Verification items for this drawing (mm, ordinates from the low corner). Round coordinates to 2 decimals unless told otherwise and drop trailing zeros. Loops run counter-clockwise (first coordinate to the right, second up) from the corner with the lowest first, then second, coordinate; pieces in that order, holes last. Notation, with made-up numbers: (46.5, 66) -> (74.5, 66) arc R17 cw to (74.5, 93) -> close; hole circle Ø2 at (-20.5, -18.75). An arc over 180 degrees is marked (long way). Use a Markdown table: item, result. Add a question column.
Q1. Sectioned sample at B-B, the plane z = 27.5. Enter the section's corners in (x, y).
Q2. Release check for a two-part mould opening along X. For the marked faces 1 and 2 record: released by +X, released by -X, zero draft, split by the parting line, or undercut.
Q3. Sectioned sample at C-C, the plane y = 118. Enter the section's corners in (x, z).
Q4. Gauge pin test, flat ends, axial feed: P1, Ø2, axis at x = 7, z = 23.5, coming from the -Y side; P2, Ø1.5, axis at y = 126.5, z = 52.5, coming from the -X side; P3, Ø8, axis at x = 8.5, y = 47, coming from the +Z side; P4, Ø2.5, axis at x = 52.5, y = 125, coming from the +Z side. Record the tip position at first contact, or that the pin passes through.
Q5. Sectioned sample at A-A, the plane x = 27.5. Enter the section's corners in (y, z).
Q6. Material ranges on L1, parallel to X at y = 41.5, z = 27.5; L2, parallel to Z at x = 27, y = 59; L3, parallel to Z at x = 25, y = 42, recorded low to high.
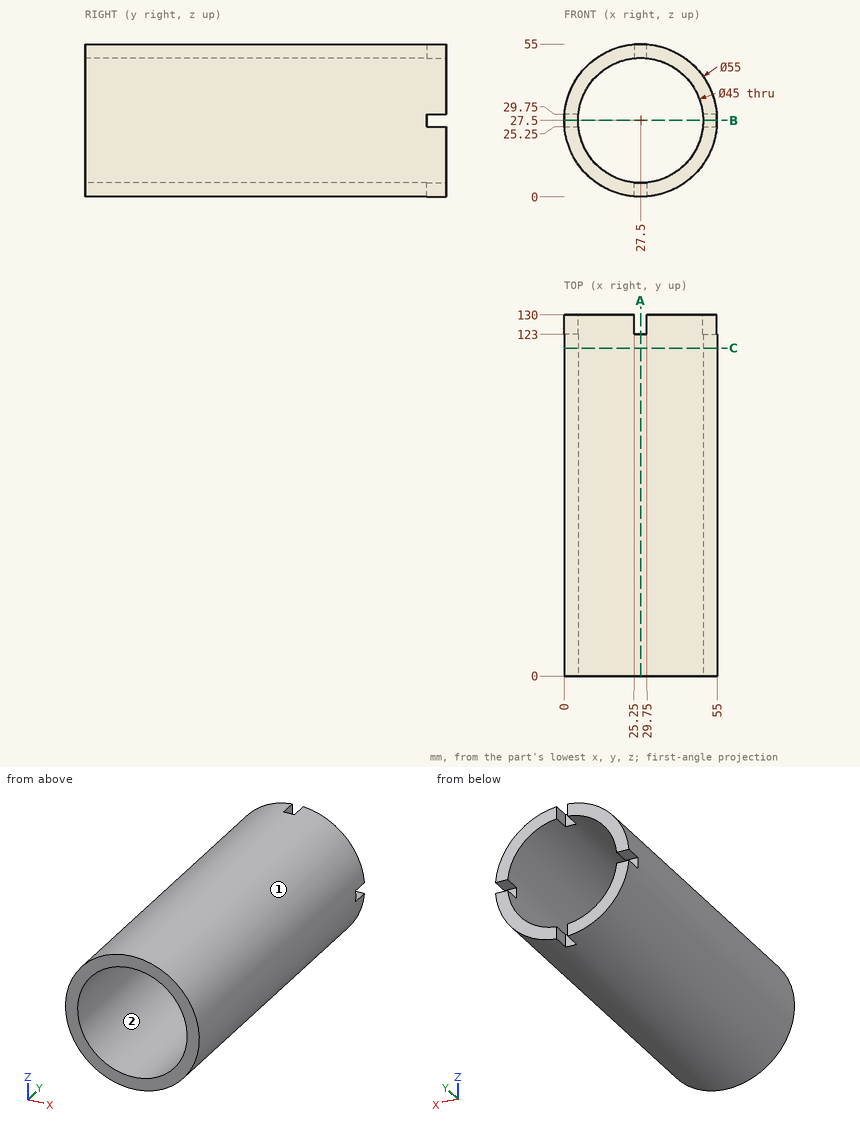
Values:
| question | item | result |
|---|---|---|
| 1 | outline | (0, 0) -> (5, 0) -> (5, 123) -> (0, 123) -> close; (50, 0) -> (55, 0) -> (55, 123) -> (50, 123) -> close |
| 2 | face 1 | split by the parting line |
| 2 | face 2 | undercut |
| 3 | outline | circle Ø55 at (27.5, 27.5); hole circle Ø45 at (27.5, 27.5) |
| 4 | P1 | through |
| 4 | P2 | x = 14.53 |
| 4 | P3 | z = 50.55 |
| 4 | P4 | z = 41.36 |
| 5 | outline | (0, 0) -> (123, 0) -> (123, 5) -> (0, 5) -> close; (0, 50) -> (123, 50) -> (123, 55) -> (0, 55) -> close |
| 6 | L1 | 0 to 5, 50 to 55 |
| 6 | L2 | 0 to 5.01, 49.99 to 55 |
| 6 | L3 | 0.11 to 5.14, 49.86 to 54.89 |
